from build123d import *

# Parameters (mm, degrees)
SKETCH1_R           = 190
SKETCH1_R_2         = 140
BOSS_EXTRUDE1_DEPTH = 75
FILLET2_R           = 20
SHELL1_T            = -2


with BuildPart() as part:
    # Sketch1 → Boss-Extrude1 (new, symmetric)
    with BuildSketch(Plane.XY):
        Circle(SKETCH1_R)
        Circle(SKETCH1_R_2, mode=Mode.SUBTRACT)
    extrude(amount=BOSS_EXTRUDE1_DEPTH, both=True)

    # Fillet2
    fillet2_edges = [part.edges().sort_by_distance(p)[0] for p in [
        (-190, 0, -75),
        (-190, 0, 75),
    ]]
    fillet(fillet2_edges, radius=FILLET2_R)

    # Shell1
    shell1_openings = [part.faces().sort_by_distance(p)[0] for p in [
        (-140, 0, 0),
    ]]
    offset(amount=SHELL1_T, openings=shell1_openings, kind=Kind.INTERSECTION)


solid = part.part
Work out the finished part from the listing and answer in its coordinate system (mm). A direction names the side the tool comes from. Round coordinates to 2 decimals unless told otherwise and drop trailing zeros. Order: outer loops, then holes, each group sorted by start corner. A loop starts at its lowest first (then second) coordinate and runs counter-clockwise, first axis right, second up. Notation, with made-up numbers: M 77.5,67.25 L 102.5,67.25 A16 ccw 102.5,71.25 Z; hole C -29.75,30 d1. An arc over 180 degrees is marked long. Put each result on its own line as item: value. Start each with the question number.
Q1. A tool of negligible diameter and unlimited length cuts with its end or side. For faces 4 (the flat face through (24, 139, -73)), 5 (the cylindrical face through (-111.1, -85.19, -74.01)), from which of +Z, -Z, +X, -X, +Y, -Y can it reach the whole face along a straight path? Write none if from no direction.
Q2. Section D-D, the plane z = -61 is taken. Write down the section's boundary in (x, y).
Q3. Section C-C, the plane z = 28 is taken. Write down the section's boundary in (x, y), and give its area (3 significant figures).
Q4. Flat-ended cylindrical pins translate along their axes: pin 1 (4 mm diameter, centred on x = -90.5, z = 43, fed in from -Y); pin 2 (12 mm diameter, centred on x = -132, y = -3.5, fed in from -Z); pin 3 (1 mm diameter, centred on x = 46.5, z = -45, fed in from -Y); pin 4 (10 mm diameter, centred on y = -49, z = -1, fed in from +X). Find the tip coordinate at first contact, or state that the pin passes through.
Q5. Straight lines are drawn through the part: L1, parallel to Z at x = -94, y = 115; L2, parallel to Y at x = 0, z = -23; L3, parallel to Y at x = -165, z = -57.5. For each, find the intervals that lie inside material, in ascending order. Write a range as [from, to].
Q6. Section A-A, the plane y = 0 is taken. Write down the section's boundary in (x, z), and give its area (3 significant figures).
Q7. For a pull along Y with two mould halves and no side action, classify faces 1 (the cylindrical face through (-111.1, -85.19, 73.99)), 2 (the flat face through (24, 139, 75)), 3 (the cylindrical face through (-41.19, -185.48, 0.77)) as pulls with the +Y half, pulls with the -Y half, needs draft (parallel to the pull), parting line crosses it, or undercut.
Findings below:
1. face 4: none
1. face 5: +Z, -Z
2. outline: C 0,0 d378.16; hole C 0,0 d373.94
3. outline: C 0,0 d380; hole C 0,0 d376
3. area: 2,380 mm^2
4. pin 1: stops at y = -168.13
4. pin 2: passes through
4. pin 3: stops at y = -184.35
4. pin 4: stops at x = 184.84
5. L1: z = [-75, -73], [73, 75]
5. L2: y = [-190, -188], [188, 190]
5. L3: y = [-93.89, -89.74], [89.74, 93.89]
6. outline: M -190,-55 A20 ccw -170,-75 L -140,-75 L -140,-73 L -170,-73 A18 cw -188,-55 L -188,55 A18 cw -170,73 L -140,73 L -140,75 L -170,75 A20 ccw -190,55 Z; M 140,-75 L 170,-75 A20 ccw 190,-55 L 190,55 A20 ccw 170,75 L 140,75 L 140,73 L 170,73 A18 cw 188,55 L 188,-55 A18 cw 170,-73 L 140,-73 Z
6. area: 919 mm^2
7. face 1: undercut
7. face 2: needs draft
7. face 3: parting line crosses it
